Read the model definition and answer for the solid it produces. Units are mm, in the model's axes. Face numbers are marked on the shaded views. A direction names the side the tool comes from. Coordinates: 2 decimals unless noted, no trailing zeros. Write each loop counter-clockwise with the first axis right and the second up, starting at its lowest first coordinate (ties: lowest second). Pieces come first, ordered by that corner, then holes.
(1) Determine the mould class of the marked faces 5, 6 and 7 for opening direction X: pulls with the +X half, pulls with the -X half, needs draft (parallel to the pull), parting line crosses it, or undercut.
(2) The part is cut by section A-A, the plane y = -16. Determine the outline of the cut face in (x, z), and give its area (3 significant figures).
(3) The part is cut by section D-D, the plane y = -19.25. Determine the outline of the cut face in (x, z).
(4) Given pin 1 (4 mm diameter, centred on y = -15.5, z = 3, fed in from -X); pin 2 (1.9 mm diameter, centred on x = 22.5, z = 4.5, fed in from -Y); pin 3 (1 mm diameter, centred on y = -18.5, z = 4.5, fed in from -X); pin 4 (1.3 mm diameter, centred on x = 17.5, z = -0.5, fed in from +Y), each flat-ended and moving along its own axis, determine where each tip first touches the part or whether it passes through.
(5) Straight lines are drawn through the part: line 1 along Z through (x, y) = (7.5, -24); line 2 along X through (y, z) = (-26.5, -4.75); line 3 along Y through (x, z) = (31, -1.25). For each, find the intervals that lie inside material, in ascending order.
(6) Which of the six approach directions +Z, -Z, +X, -X, +Y, -Y give full straight-line access (tool end or side, diameter ignored) to the marked faces 1, 2, 3 and 4?
(7) The part is cut by section C-C, the plane x = 36. Determine the outline of the cut face in (y, z), and give its area (3 significant figures).
(8) The part is cut by section B-B, the plane z = -1. Determine the outline of the cut face in (x, y).
```python
from build123d import *

# Parameters (mm, degrees)
F1_DEPTH  = 1.6002
F2_W      = 37.084
F2_H      = 20.701
F3_DEPTH  = 3.81
F4_W      = 7.7978
F4_H      = 3.2512
F5_DEPTH  = 2.1209
F6_R      = 0.508
F7_DEPTH  = 25.4
F8_W      = 6.35
F8_H      = 16.51
F9_DEPTH  = 7.9502
F10_W     = 7.62
F10_H     = 8.128
F11_DEPTH = 5.8674
F12_W     = 23.876
F12_H     = 3.81
F13_DEPTH = 1.5875
F14_W     = 8.128
F14_H     = 5.4737
F14_H_2   = 4.1275
F15_DEPTH = 3.048
F16_W     = 34.6964
F16_H     = 18.796
F16_W_2   = 23.876
F16_H_2   = 3.81
F17_DEPTH = 5.3086


with BuildPart() as f1:
    # F0 (on Top) → F1 (new body)
    with BuildSketch(Plane.XY):
        with BuildLine():
            Line((37.2917920684, -4.2399411205), (-3.3482079316, -4.2399411205))
            Line((-3.3482079316, -4.2399411205), (-3.3482079316, -27.6079411205))
            ThreePointArc((-3.3482079316, -27.6079411205), (-2.4501657042, -30.6373636727), (-0.0462079316, -32.6879411205))
            Line((-0.0462079316, -32.6879411205), (40.5937920684, -32.6879411205))
            Line((40.5937920684, -32.6879411205), (40.5937920684, -9.3199411205))
            ThreePointArc((40.5937920684, -9.3199411205), (39.6957498411, -6.2905185683), (37.2917920684, -4.2399411205))
        make_face()
    extrude(amount=F1_DEPTH)

    # F2 (on face) → F3 (join)
    with BuildSketch(Plane.XY.offset(1.6002)):
        with Locations((18.4957920684, -17.4098411205)):
            Rectangle(F2_W, F2_H)
    extrude(amount=F3_DEPTH)

    # F4 (on face) → F5 (join)
    with BuildSketch(Plane(origin=(-0.0462079316, 0, 0), x_dir=(0, -1, 0), z_dir=(-1, 0, 0))):
        with Locations((17.8162411205, 3.7846)):
            Rectangle(F4_W, F4_H)
    extrude(amount=F5_DEPTH)

    # F6 (on face) → F7 (cut)
    with BuildSketch(Plane.XY.offset(1.6002)):
        with Locations((6.5577920684, -30.3003411205)):
            Circle(F6_R)
        with Locations((9.0977920684, -30.3003411205)):
            Circle(F6_R)
        with Locations((11.6377920684, -30.3003411205)):
            Circle(F6_R)
    extrude(amount=-F7_DEPTH, mode=Mode.SUBTRACT)

    # F8 (on face) → F9 (join)
    with BuildSketch(Plane(origin=(0, 0, 0), x_dir=(1, 0, 0), z_dir=(0, 0, -1))):
        with Locations((1.8587920684, 22.6549411205)):
            Rectangle(F8_W, F8_H)
    extrude(amount=F9_DEPTH)

    # F10 (on face) → F11 (join)
    with BuildSketch(Plane(origin=(0, 0, 0), x_dir=(1, 0, 0), z_dir=(0, 0, -1))):
        with Locations((2.4937920684, 9.4723411205)):
            Rectangle(F10_W, F10_H)
    extrude(amount=F11_DEPTH)

    # F12 (on face) → F13 (join)
    with BuildSketch(Plane(origin=(0, 0, 0), x_dir=(1, 0, 0), z_dir=(0, 0, -1))):
        with Locations((20.4515920684, 19.0989411205)):
            Rectangle(F12_W, F12_H)
    extrude(amount=F13_DEPTH)

    # F14 (on face) → F15 (join)
    with BuildSketch(Plane(origin=(0, 0, 0), x_dir=(1, 0, 0), z_dir=(0, 0, -1))):
        with Locations((27.4492920684, 5.6305911205)):
            Rectangle(F14_W, F14_H)
        with Locations((27.4492920684, 6.3036911205)):
            Rectangle(F14_W, F14_H_2)
    extrude(amount=F15_DEPTH)

    # F16 (on face) → F17 (join)
    with BuildSketch(Plane(origin=(0, 0, -1.5875), x_dir=(1, 0, 0), z_dir=(0, 0, -1))):
        with Locations((23.2455920684, 23.2899411205)):
            Rectangle(F16_W, F16_H)
        with Locations((20.4515920684, 19.0989411205)):
            Rectangle(F16_W_2, F16_H_2, mode=Mode.SUBTRACT)
        with Locations((23.2455920684, 23.2899411205)):
            Rectangle(F16_W, F16_H)
    extrude(amount=F17_DEPTH)


solid = f1.part
```
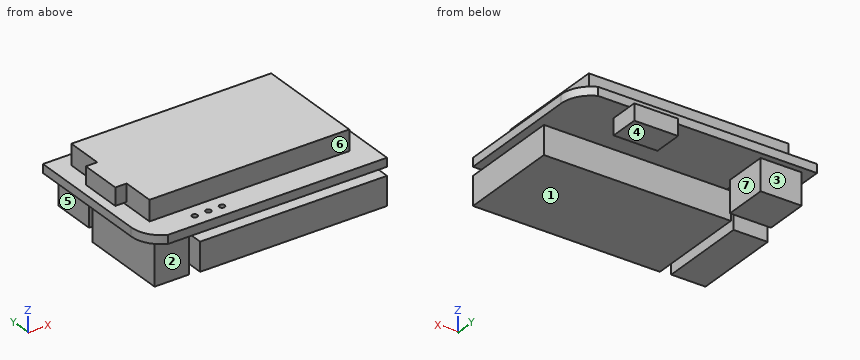
Computed:
1. face 5: pulls with the -X half
1. face 6: needs draft
1. face 7: undercut
2. outline: (-3.35, 0) - (-1.32, 0) - (-1.32, -7.95) - (5.03, -7.95) - (5.03, 0) - (40.59, 0) - (40.59, 1.6) - (37.04, 1.6) - (37.04, 5.41) - (-2.17, 5.41) - (-2.17, 2.16) - (-0.05, 2.16) - (-0.05, 1.6) - (-3.35, 1.6) - close; (5.9, -6.9) - (40.59, -6.9) - (40.59, -1.59) - (5.9, -1.59) - close
2. area: 453 mm2
3. outline: (-3.35, 0) - (-1.32, 0) - (-1.32, -7.95) - (5.03, -7.95) - (5.03, 0) - (8.51, 0) - (8.51, -1.59) - (5.9, -1.59) - (5.9, -6.9) - (40.59, -6.9) - (40.59, -1.59) - (32.39, -1.59) - (32.39, 0) - (40.59, 0) - (40.59, 1.6) - (37.04, 1.6) - (37.04, 5.41) - (-2.17, 5.41) - (-2.17, 2.16) - (-0.05, 2.16) - (-0.05, 1.6) - (-3.35, 1.6) - close
4. pin 1: stops at x = -3.35
4. pin 2: stops at y = -27.76
4. pin 3: stops at x = -2.17
4. pin 4: stops at y = -4.24
5. line 1: z = -6.9 to -1.59, 0 to 5.41
5. line 2: x = -1.32 to 5.03, 5.9 to 40.59
5. line 3: y = -21 to -17.19, -8.37 to -2.89
6. face 1: -Z, +X, +Y, -Y
6. face 2: -Z, -X, -Y
6. face 3: -Z, -X, +Y
6. face 4: -Z, +X, +Y
7. outline: (-32.69, -6.9) - (-13.89, -6.9) - (-13.89, -1.59) - (-32.69, -1.59) - close; (-32.69, 0) - (-4.24, 0) - (-4.24, 1.6) - (-7.06, 1.6) - (-7.06, 5.41) - (-27.76, 5.41) - (-27.76, 1.6) - (-32.69, 1.6) - close
7. area: 224 mm2
8. outline: (-1.32, -30.91) - (5.03, -30.91) - (5.03, -14.4) - (-1.32, -14.4) - close; (-1.32, -13.54) - (6.3, -13.54) - (6.3, -5.41) - (-1.32, -5.41) - close; (8.51, -21) - (32.39, -21) - (32.39, -17.19) - (8.51, -17.19) - close; (23.39, -8.37) - (31.51, -8.37) - (31.51, -2.89) - (23.39, -2.89) - close
